For this review, take the finished solid that the model builds, in its own axes (mm). Face numbers are marked on the shaded views. A direction names the side the tool comes from. Round coordinates to 2 decimals unless told otherwise and drop trailing zeros. Loops run counter-clockwise (first coordinate to the right, second up) from the corner with the lowest first, then second, coordinate; pieces in that order, holes last.
1) Take a section at B-B (z = 0). State the section outline as (x, y) points.
2) Take a section at C-C (x = 15). State the section outline as (y, z) points, then the cut area to 3 significant figures.
3) Take a section at D-D (y = -30.5). State the section outline as (x, z) points, then the cut area to 3 significant figures.
4) Mouldability with a two-part tool opening along Z and no side actions: class the marked faces 4, 5 and 6 as pulls with the +Z half, pulls with the -Z half, needs draft (parallel to the pull), parting line crosses it, or undercut.
5) Wall thickness on L1, parallel to Z at x = -12, y = 0; L2, parallel to Y at x = -10.5, z = -1; L3, parallel to X at y = 41.5, z = -2: over which ranges is each line inside the solid? List them lowest first.
6) Take a section at A-A (y = 0). State the section outline as (x, z) points, then the cut area to 3 significant figures.
7) Insertion check: pin 1 (20.5 mm diameter, centred on y = 0, z = 0, fed in from +X); pin 2 (1.5 mm diameter, centred on x = -1, y = 18, fed in from +Z); pin 3 (13.5 mm diameter, centred on y = -1.5, z = -30.5, fed in from -X). Each pin has a flat end and moves straight along its axis. Give the tip position at first contact, or say it passes through.
8) Tool access review of the marked faces 1, 2 and 3: name each direction out of +Z, -Z, +X, -X, +Y, -Y from which nothing blocks a thin tool from reaching the whole face with its end or side.
```python
from build123d import *

# Parameters (mm, degrees)
F0_W     = 12
F0_H     = 35.9999971587
F2_R     = 8.3712602983
F3_DEPTH = 5


with BuildPart() as f1:
    # F0 (on Top) → F1 (revolve)
    with BuildSketch(Plane.XY):
        Polygon((-19.4594625823, 44.9189218498), (-6.4864925787, 44.9189218498), (5.5135074213, 44.9189218498), (19.1351225156, 44.9189218498), (19.1351225156, 56.9189218498), (-19.4594625823, 56.9189218498), align=None)
        with Locations((-0.4864925787, 26.9189232705)):
            Rectangle(F0_W, F0_H)
    revolve(axis=Axis((2.7567485016, 0, 0), (1, 0, 0)))

    # F2 (on face) → F3 (join)
    with BuildSketch(Plane(origin=(-6.4864925787, 0, 0), x_dir=(0, -1, 0), z_dir=(-1, 0, 0))):
        with Locations((0, 27.9054697603)):
            Circle(F2_R)
        with Locations((0, -27.5865457952)):
            Circle(F2_R)
    extrude(amount=F3_DEPTH)


solid = f1.part
```
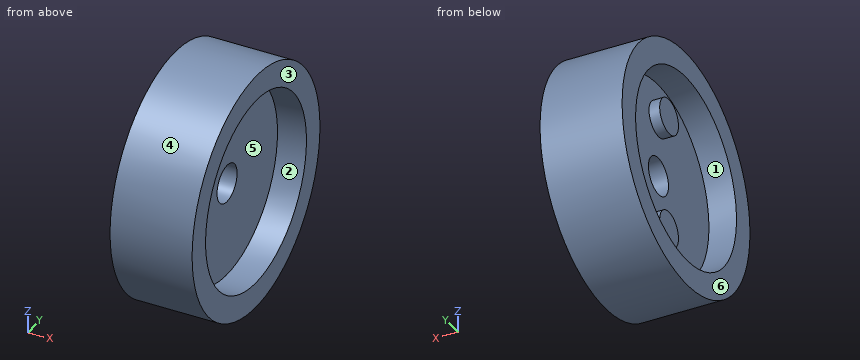
Response:
1. outline: (-19.46, -56.92) - (19.14, -56.92) - (19.14, -44.92) - (5.51, -44.92) - (5.51, -8.92) - (-6.49, -8.92) - (-6.49, -44.92) - (-19.46, -44.92) - close; (-19.46, 44.92) - (-6.49, 44.92) - (-6.49, 8.92) - (5.51, 8.92) - (5.51, 44.92) - (19.14, 44.92) - (19.14, 56.92) - (-19.46, 56.92) - close
2. outline: circle Ø113.84 at (0, 0); hole circle Ø89.84 at (0, 0)
2. area: 3,840 mm2
3. outline: (-19.46, -48.06) - (19.14, -48.06) - (19.14, -32.98) - (5.51, -32.98) - (5.51, 32.98) - (19.14, 32.98) - (19.14, 48.06) - (-19.46, 48.06) - (-19.46, 32.98) - (-6.49, 32.98) - (-6.49, -32.98) - (-19.46, -32.98) - close
3. area: 1,960 mm2
4. face 4: parting line crosses it
4. face 5: undercut
4. face 6: needs draft
5. L1: z = -56.92 to -44.92, 44.92 to 56.92
5. L2: y = -56.91 to -44.91, 44.91 to 56.91
5. L3: x = -6.49 to 5.51
6. outline: (-19.46, -56.92) - (19.14, -56.92) - (19.14, -44.92) - (5.51, -44.92) - (5.51, -8.92) - (-6.49, -8.92) - (-6.49, -19.22) - (-11.49, -19.22) - (-11.49, -35.96) - (-6.49, -35.96) - (-6.49, -44.92) - (-19.46, -44.92) - close; (-19.46, 44.92) - (-6.49, 44.92) - (-6.49, 36.28) - (-11.49, 36.28) - (-11.49, 19.53) - (-6.49, 19.53) - (-6.49, 8.92) - (5.51, 8.92) - (5.51, 44.92) - (19.14, 44.92) - (19.14, 56.92) - (-19.46, 56.92) - close
6. area: 1,960 mm2
7. pin 1: stops at x = 5.51
7. pin 2: stops at z = 54.24
7. pin 3: stops at x = -11.49
8. face 1: -X
8. face 2: +X
8. face 3: +Z, -Z, +X, +Y, -Y
